Geometry: final body of the model. Coordinates: model frame, mm. Round coordinates to 2 decimals unless told otherwise and drop trailing zeros. Loops run counter-clockwise (first coordinate to the right, second up) from the corner with the lowest first, then second, coordinate; pieces in that order, holes last. Notation, with made-up numbers: (51.25, -11) - (87.25, -11) arc R17 cw to (87.25, 5) - close; hole circle Ø4 at (-14, 20.25). An arc over 180 degrees is marked (long way). Return JSON: item names as keys, results as strings. Group by question number.
1. Draft query along X for faces 1 (the face through (24.65, 2.46, -9.72)), 2 (the face through (0, 0, -3)), 3 (the face through (-24.65, 2.46, 9.72)), 4 (the face through (0, 2, -2.4)). Return one class per face: +X half, -X half, draft (parallel to the pull), parting line (faces both ways), or undercut.
2. Material intervals for probe 1 along X at (y, z) = (3.4, 0); probe 2 along Z at (x, y) = (0.5, 2.9); probe 3 along X at (y, z) = (2.8, 0.5) (3 decimals), sorted ascending.
3. First-contact query: pin 1 Ø1.5 at (y, z) = (3, -4) entering from -X. Flat tip, straight axial feed; report the tip coordinate or a pass-through.
4. Section D-D on x = -22.5. Return loops of the section in (y, z), and give its area (3 significant figures).
5. Section B-B on x = 0. Return loops of the section in (y, z), and give its area (3 significant figures).
6. Section C-C on y = 2.4. Return loops of the section in (x, z).
7. Section A-A on z = 0. Return loops of the section in (x, y), and give its area (3 significant figures).
from build123d import *

# Parameters (mm, degrees)
SZKIC1_R                    = 2.3
DODANIE_WYCI_GNI_CIE1_DEPTH = 5


with BuildPart() as part:
    # Szkic1 → Dodanie-wyciągnięcie1 (new body)
    with BuildSketch(Plane(origin=(0, 0, 0), x_dir=(1, 0, 0), z_dir=(0, 1, 0))):
        with BuildLine():
            Line((-17.5, -12.72606383), (17.5, -12.72606383))
            ThreePointArc((17.5, -12.72606383), (24.571067812, -9.797131642), (27.5, -2.72606383))
            Line((27.5, -2.72606383), (27.5, 2.72606383))
            ThreePointArc((27.5, 2.72606383), (24.571067812, 9.797131642), (17.5, 12.72606383))
            Line((17.5, 12.72606383), (-17.5, 12.72606383))
            ThreePointArc((-17.5, 12.72606383), (-24.571067812, 9.797131642), (-27.5, 2.72606383))
            Line((-27.5, 2.72606383), (-27.5, -2.72606383))
            ThreePointArc((-27.5, -2.72606383), (-24.571067812, -9.797131642), (-17.5, -12.72606383))
        make_face()
        with Locations(Location((-22.5, 0, 0), (0, 0, 270))):
            Circle(SZKIC1_R, mode=Mode.SUBTRACT)
        with Locations(Location((22.5, 0, 0), (0, 0, 90))):
            Circle(SZKIC1_R, mode=Mode.SUBTRACT)
        with BuildLine():
            Line((-1.8, 2.4), (1.8, 2.4))
            ThreePointArc((1.8, 2.4), (0, -3), (-1.8, 2.4))
        make_face(mode=Mode.SUBTRACT)
    extrude(amount=DODANIE_WYCI_GNI_CIE1_DEPTH)


solid = part.part
Taken from the geometry:
{
 "1": {"face 1": "+X half", "face 2": "draft", "face 3": "-X half", "face 4": "undercut"},
 "2": {"probe 1": "-27.5 to -24.8, -20.2 to -3, 3 to 20.2, 24.8 to 27.5", "probe 2": "-12.73 to -2.4, 2.96 to 12.73", "probe 3": "-27.5 to -24.745, -20.255 to -2.958, 2.958 to 20.255, 24.745 to 27.5"},
 "3": {"pin 1": "x = -27.49"},
 "4": {"outline": "(0, -11.39) - (5, -11.39) - (5, -2.3) - (0, -2.3) - close; (0, 2.3) - (5, 2.3) - (5, 11.39) - (0, 11.39) - close", "area": "90.9 mm2"},
 "5": {"outline": "(0, -12.73) - (5, -12.73) - (5, -2.4) - (0, -2.4) - close; (0, 3) - (5, 3) - (5, 12.73) - (0, 12.73) - close", "area": "100 mm2"},
 "6": {"outline": "(-27.5, -2.73) arc R10 ccw to (-17.5, -12.73) - (17.5, -12.73) arc R10 ccw to (27.5, -2.73) - (27.5, 2.73) arc R10 ccw to (17.5, 12.73) - (-17.5, 12.73) arc R10 ccw to (-27.5, 2.73) - close; hole circle Ø4.6 at (-22.5, 0); hole (-1.8, -2.4) - (1.8, -2.4) arc R3 ccw (long way) to start; hole circle Ø4.6 at (22.5, 0)"},
 "7": {"outline": "(-27.5, 0) - (-24.8, 0) - (-24.8, 5) - (-27.5, 5) - close; (-20.2, 0) - (-3, 0) - (-3, 5) - (-20.2, 5) - close; (3, 0) - (20.2, 0) - (20.2, 5) - (3, 5) - close; (24.8, 0) - (27.5, 0) - (27.5, 5) - (24.8, 5) - close", "area": "199 mm2"}
}
